```python
from build123d import *

# Parameters (mm, degrees)
BOX_W         = 10
BOX_H         = 106
BOX_DEPTH     = 1
EXTRUDE_DEPTH = 10


with BuildPart() as cube:
    # Box → Box (new body)
    with BuildSketch(Plane(origin=(-6, -53, 0), x_dir=(1, 0, 0), z_dir=(0, 0, 1))):
        with Locations((5, 53)):
            Rectangle(BOX_W, BOX_H)
    extrude(amount=BOX_DEPTH)


with BuildPart() as fusion:
    # Offset2D → Extrude (new body)
    with BuildSketch(Plane(origin=(-0.426228, -0.837563, 0), x_dir=(0, 1, 0), z_dir=(0, 0, 1))):
        with BuildLine():
            ThreePointArc((42.503525, -24.276272), (49.68176, -13.31089), (52.080118, -0.426228))
            ThreePointArc((52.080118, -0.426228), (51.015355, 5.810333), (48.264258, 11.507689))
            ThreePointArc((48.264258, 11.507689), (43.784533, 18.605601), (38.309512, 24.967395))
            ThreePointArc((38.309512, 24.967395), (31.855149, 29.634938), (24.288431, 32.122818))
            ThreePointArc((24.288431, 32.122818), (16.786489, 31.750925), (9.812264, 28.962088))
            ThreePointArc((9.812264, 28.962088), (5.058836, 25.712847), (0.837563, 21.797045))
            ThreePointArc((0.837563, 21.797045), (-3.138279, 25.368097), (-7.109626, 28.944146))
            ThreePointArc((-7.109626, 28.944146), (-12.158639, 32.433141), (-17.702089, 35.066729))
            ThreePointArc((-17.702089, 35.066729), (-24.054754, 35.79826), (-30.365509, 34.765847))
            ThreePointArc((-30.365509, 34.765847), (-39.957434, 27.594753), (-46.857377, 17.805962))
            ThreePointArc((-46.857377, 17.805962), (-50.317164, 6.059483), (-49.039004, -6.11903))
            ThreePointArc((-49.039004, -6.11903), (-44.500868, -17.280695), (-37.495914, -27.084166))
            ThreePointArc((-37.495914, -27.084166), (-25.986015, -34.811524), (-12.196241, -36.236991))
            ThreePointArc((-12.196241, -36.236991), (-5.835332, -34.400867), (-0.433382, -30.573144))
            ThreePointArc((-0.433382, -30.573144), (4.594591, -24.567416), (9.422656, -18.399834))
            ThreePointArc((9.422656, -18.399834), (12.730523, -21.735725), (16.175134, -24.930222))
            ThreePointArc((16.175134, -24.930222), (29.464589, -29.646272), (42.503525, -24.276272))
        make_face()
        with BuildLine():
            ThreePointArc((50.580413, -0.458151), (48.292873, -12.744264), (41.45398, -23.204232))
            ThreePointArc((41.45398, -23.204232), (29.420995, -28.146891), (17.160495, -23.799162))
            ThreePointArc((17.160495, -23.799162), (13.767835, -20.652193), (10.509658, -17.366187))
            ThreePointArc((10.509658, -17.366187), (9.338332, -16.902206), (8.226493, -17.49474))
            ThreePointArc((8.226493, -17.49474), (3.446379, -23.60181), (-1.530981, -29.549219))
            ThreePointArc((-1.530981, -29.549219), (-6.510376, -33.061053), (-12.365823, -34.746608))
            ThreePointArc((-12.365823, -34.746608), (-12.386537, -34.749111), (-12.407214, -34.751901))
            ThreePointArc((-12.407214, -34.751901), (-25.475718, -33.400993), (-36.383595, -26.077812))
            ThreePointArc((-36.383595, -26.077812), (-36.384661, -26.076636), (-36.385727, -26.075461))
            ThreePointArc((-36.385727, -26.075461), (-43.186869, -16.557226), (-47.592966, -5.720316))
            ThreePointArc((-47.592966, -5.720316), (-47.599325, -5.69793), (-47.606032, -5.675645))
            ThreePointArc((-47.606032, -5.675645), (-48.823362, 5.923269), (-45.528232, 17.11071))
            ThreePointArc((-45.528232, 17.11071), (-45.519523, 17.12762), (-45.511029, 17.144638))
            ThreePointArc((-45.511029, 17.144638), (-38.930567, 26.499036), (-29.789964, 33.373381))
            ThreePointArc((-29.789964, 33.373381), (-23.99136, 34.299325), (-18.157006, 33.634866))
            ThreePointArc((-18.157006, 33.634866), (-12.888907, 31.122689), (-8.086797, 27.805513))
            ThreePointArc((-8.086797, 27.805513), (-4.127663, 24.240509), (-0.164064, 20.680469))
            ThreePointArc((-0.164064, 20.680469), (0.905659, 20.298592), (1.936336, 20.77592))
            ThreePointArc((1.936336, 20.77592), (5.994706, 24.540606), (10.564694, 27.664456))
            ThreePointArc((10.564694, 27.664456), (10.577868, 27.672185), (10.590962, 27.680047))
            ThreePointArc((10.590962, 27.680047), (17.089081, 30.281647), (24.079619, 30.636968))
            ThreePointArc((24.079619, 30.636968), (31.187217, 28.29176), (37.251055, 23.904526))
            ThreePointArc((37.251055, 23.904526), (42.579895, 17.711815), (46.940184, 10.802829))
            ThreePointArc((46.940184, 10.802829), (46.977469, 10.736863), (47.018038, 10.672863))
            ThreePointArc((47.018038, 10.672863), (49.584915, 5.358808), (50.580413, -0.458151))
        make_face(mode=Mode.SUBTRACT)
        with BuildLine():
            ThreePointArc((35.552622, 15.131092), (33.338518, 16.701666), (30.923044, 17.940394))
            ThreePointArc((30.923044, 17.940394), (27.946256, 18.236801), (25.105466, 17.299229))
            ThreePointArc((25.105466, 17.299229), (23.967442, 15.978028), (22.837721, 14.649721))
            ThreePointArc((22.837721, 14.649721), (17.31029, 5.569336), (12.663486, -3.991684))
            ThreePointArc((12.663486, -3.991684), (11.790559, -8.016187), (13.080744, -11.926946))
            ThreePointArc((13.080744, -11.926946), (16.552966, -14.14054), (20.476526, -15.390342))
            ThreePointArc((20.476526, -15.390342), (24.918231, -14.563002), (28.821685, -12.287857))
            ThreePointArc((28.821685, -12.287857), (35.396432, -2.057673), (38.294161, 9.752794))
            ThreePointArc((38.294161, 9.752794), (37.823131, 12.900577), (35.552622, 15.131092))
        make_face()
        with BuildLine():
            ThreePointArc((30.40309, 16.531325), (32.591653, 15.400263), (34.599518, 13.972822))
            ThreePointArc((34.599518, 13.972822), (34.741804, 13.86912), (34.895262, 13.782805))
            ThreePointArc((34.895262, 13.782805), (36.486738, 12.219363), (36.816899, 10.012976))
            ThreePointArc((36.816899, 10.012976), (36.80583, 9.939531), (36.798411, 9.865628))
            ThreePointArc((36.798411, 9.865628), (34.038666, -1.417946), (27.779717, -11.203691))
            ThreePointArc((27.779717, -11.203691), (24.416076, -13.149361), (20.601053, -13.887812))
            ThreePointArc((20.601053, -13.887812), (17.225415, -12.799054), (14.217244, -10.919895))
            ThreePointArc((14.217244, -10.919895), (13.283803, -7.831341), (13.99417, -4.683985))
            ThreePointArc((13.99417, -4.683985), (14.019039, -4.633927), (14.042025, -4.582977))
            ThreePointArc((14.042025, -4.582977), (18.607638, 4.815324), (24.035661, 13.743338))
            ThreePointArc((24.035661, 13.743338), (25.047691, 14.93331), (26.066422, 16.11755))
            ThreePointArc((26.066422, 16.11755), (28.193734, 16.754377), (30.40309, 16.531325))
        make_face(mode=Mode.SUBTRACT)
        with BuildLine():
            ThreePointArc((-5.304279, 16.390724), (-8.42234, 18.854547), (-11.956744, 20.671333))
            ThreePointArc((-11.956744, 20.671333), (-17.494369, 20.574952), (-22.66759, 18.596983))
            ThreePointArc((-22.66759, 18.596983), (-31.070315, 10.860543), (-37.498867, 1.41957))
            ThreePointArc((-37.498867, 1.41957), (-39.844627, -4.40289), (-40.673419, -10.625168))
            ThreePointArc((-40.673419, -10.625168), (-38.087415, -15.735136), (-33.892074, -19.633635))
            ThreePointArc((-33.892074, -19.633635), (-30.444372, -21.380497), (-26.661131, -22.171232))
            ThreePointArc((-26.661131, -22.171232), (-19.969831, -20.610018), (-14.438078, -16.534407))
            ThreePointArc((-14.438078, -16.534407), (-7.758227, -5.295928), (-3.155024, 6.94067))
            ThreePointArc((-3.155024, 6.94067), (-2.90689, 11.966537), (-5.304279, 16.390724))
        make_face()
        with BuildLine():
            ThreePointArc((-12.354501, 19.214576), (-9.175054, 17.555033), (-6.363544, 15.328291))
            ThreePointArc((-6.363544, 15.328291), (-4.366665, 11.621196), (-4.577792, 7.415782))
            ThreePointArc((-4.577792, 7.415782), (-4.589381, 7.379554), (-4.600048, 7.343045))
            ThreePointArc((-4.600048, 7.343045), (-9.092234, -4.608778), (-15.606542, -15.590107))
            ThreePointArc((-15.606542, -15.590107), (-20.599769, -19.248702), (-26.624616, -20.669563))
            ThreePointArc((-26.624616, -20.669563), (-29.983258, -19.952576), (-33.044569, -18.396002))
            ThreePointArc((-33.044569, -18.396002), (-33.062278, -18.38406), (-33.080155, -18.372371))
            ThreePointArc((-33.080155, -18.372371), (-36.821301, -14.922254), (-39.17073, -10.407872))
            ThreePointArc((-39.17073, -10.407872), (-38.364838, -4.675009), (-36.188487, 0.689566))
            ThreePointArc((-36.188487, 0.689566), (-36.179503, 0.705932), (-36.170723, 0.722409))
            ThreePointArc((-36.170723, 0.722409), (-29.95755, 9.85407), (-21.840097, 17.343912))
            ThreePointArc((-21.840097, 17.343912), (-17.257745, 19.092821), (-12.354501, 19.214576))
        make_face(mode=Mode.SUBTRACT)
    extrude(amount=EXTRUDE_DEPTH)

    # Fusion: union Cube
    add(cube.part)


solid = fusion.part
```
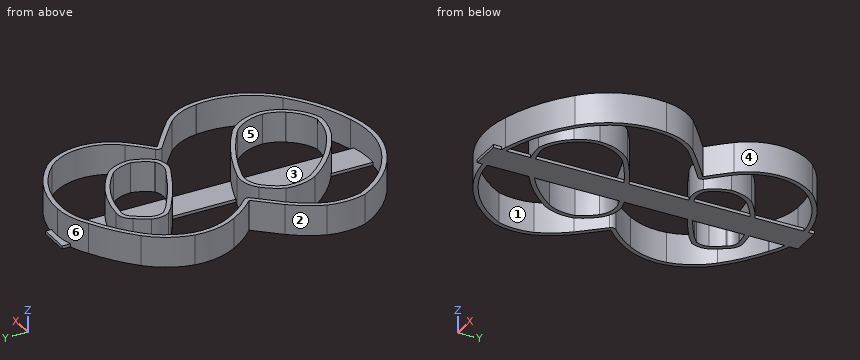
Source: CAD feature listing. Evaluate the final solid. Frame: model axes, mm. Face numbers are marked on the shaded views. A direction names the side the tool comes from. Give positions to 0.01 mm unless a question says otherwise; leave off trailing zeros. Loops run counter-clockwise (first coordinate to the right, second up) from the corner with the lowest first, then second, coordinate; pieces in that order, holes last. Notation, with made-up numbers: (-20, -1) -> (11, -1) arc R31 cw to (11, 23) -> close; hole circle Ø5 at (10.25, 86.5). An arc over 180 degrees is marked (long way). Use a Markdown table: item, result. Add a question column.
(1) Access query for the marked faces 1, 2 and 3. Directions: +Z, -Z, +X, -X, +Y, -Y. A direction counts if a zero-diameter tool reaches every point of the face in a straight line with its end or side. Return the directions, or none.
(2) Pull-direction query (X, two-part tool) for the marked faces 4, 5 and 6; classes: +X half, -X half, draft (parallel to the pull), parting line (faces both ways), or undercut.
(3) Section query B-B (z = 3). Count the separate pieces of the cut face and the enclosed holes in it, then the cut area to 3 significant figures.
(4) Ray query, line 1 (X direction, y = 21, z = 3); line 2 (Y direction, x = 1, z = 3.25); line 3 (Y direction, x = -10, z = 1.5). Return the intervals inside material, ascending.
(5) Section query A-A (y = -44). Output: boundary loops of the cut face in (x, z).
(6) First-contact query: pin 1 Ø3 at (y, z) = (-11.5, 2.5) entering from +X; pin 2 Ø4 at (x, z) = (6.5, 6) entering from +Y; pin 3 Ø1.1 at (y, z) = (-15.5, 0.5) entering from -X. Flat tips, straight axial feed; report the tip coordinate or a pass-through.
Checked values:
| question | item | result |
|---|---|---|
| 1 | face 1 | +Z, -Z |
| 1 | face 2 | +Z, -Z, -X |
| 1 | face 3 | +Z |
| 2 | face 4 | +X half |
| 2 | face 5 | undercut |
| 2 | face 6 | -X half |
| 3 | separate pieces | 3 |
| 3 | enclosed holes | 3 |
| 3 | area | 758 mm^2 |
| 4 | line 1 | -32.7 to -31.2, -13.57 to -10.78, 13.37 to 14.88, 26.27 to 27.89 |
| 4 | line 2 | -50.94 to -49.43, -39.7 to -38.07, -8.5 to -6.87, 12.96 to 14.62, 33.2 to 34.82, 49.74 to 51.24 |
| 4 | line 3 | -50.63 to -49.1, -32.98 to -31.03, -5.02 to -3.52, 18.77 to 20.52, 35.94 to 37.44, 46.87 to 48.59 |
| 5 | outline | (-24.27, 0) -> (-21.66, 0) -> (-21.66, 10) -> (-24.27, 10) -> close; (-6, 0) -> (4, 0) -> (4, 1) -> (-6, 1) -> close; (16.18, 0) -> (19.14, 0) -> (19.14, 10) -> (16.18, 10) -> close |
| 6 | pin 1 | x = 35.81 |
| 6 | pin 2 | y = 51 |
| 6 | pin 3 | x = -34.45 |
